Here's how the part is built. I have some questions about the finished solid (model axes, mm). A direction names the side the tool comes from. Coordinates: 2 decimals unless noted, no trailing zeros. Order: outer loops, then holes, each group sorted by start corner. A loop starts at its lowest first (then second) coordinate and runs counter-clockwise, first axis right, second up. Notation, with made-up numbers: (43.25, -30) -> (72.25, -30) arc R15 ccw to (72.25, -9) -> close; hole circle Ø5 at (7, 15.5). An arc over 180 degrees is marked (long way). One line per item, written item: value. Start each with the question number.
```python
from build123d import *

# Parameters (mm, degrees)
F1_DEPTH = 1.5
F2_DEPTH = 14
F4_W     = 26.8
F4_H     = 15.749622
F5_DEPTH = 26
F6_R     = 3
F7_R     = 0.7
F9_DEPTH = 18.8


with BuildPart() as f1:
    # F0 (on Top) → F1 (new body)
    with BuildSketch(Plane.XY):
        Polygon((0, -17.666918), (15.3, -8.833459), (15.3, 8.833459), (0, 17.666918), (-15.3, 8.833459), (-15.3, -8.833459), align=None)
        with BuildLine():
            ThreePointArc((-6.22254, -8.626703), (-8.626703, -8.626703), (-8.626703, -6.22254))
            Line((-8.626703, -6.22254), (-6.505382, -4.101219))
            ThreePointArc((-6.505382, -4.101219), (-4.101219, -4.101219), (-4.101219, -6.505382))
            Line((-4.101219, -6.505382), (-6.22254, -8.626703))
        make_face(mode=Mode.SUBTRACT)
        with BuildLine():
            ThreePointArc((8.626703, -6.22254), (8.626703, -8.626703), (6.22254, -8.626703))
            Line((6.22254, -8.626703), (4.101219, -6.505382))
            ThreePointArc((4.101219, -6.505382), (4.101219, -4.101219), (6.505382, -4.101219))
            Line((6.505382, -4.101219), (8.626703, -6.22254))
        make_face(mode=Mode.SUBTRACT)
        with BuildLine():
            ThreePointArc((-8.626703, 6.22254), (-8.626703, 8.626703), (-6.22254, 8.626703))
            Line((-6.22254, 8.626703), (-4.101219, 6.505382))
            ThreePointArc((-4.101219, 6.505382), (-4.101219, 4.101219), (-6.505382, 4.101219))
            Line((-6.505382, 4.101219), (-8.626703, 6.22254))
        make_face(mode=Mode.SUBTRACT)
        with BuildLine():
            Line((4.101219, 6.505382), (6.22254, 8.626703))
            ThreePointArc((6.22254, 8.626703), (8.626703, 8.626703), (8.626703, 6.22254))
            Line((8.626703, 6.22254), (6.505382, 4.101219))
            ThreePointArc((6.505382, 4.101219), (4.101219, 4.101219), (4.101219, 6.505382))
        make_face(mode=Mode.SUBTRACT)
    extrude(amount=F1_DEPTH)

    # F0 (on Top) → F2 (join)
    with BuildSketch(Plane.XY):
        Polygon((-17.8, 10.276835), (-17.8, -10.276835), (0, -20.55367), (17.8, -10.276835), (17.8, 10.276835), (0, 20.55367), align=None)
        Polygon((15.3, 8.833459), (15.3, -8.833459), (0, -17.666918), (-15.3, -8.833459), (-15.3, 8.833459), (0, 17.666918), align=None, mode=Mode.SUBTRACT)
    extrude(amount=F2_DEPTH)

    # F4 (on offset) → F5 (cut)
    with BuildSketch(Plane.XZ.offset(-25)):
        with Locations((0, 9.374811)):
            Rectangle(F4_W, F4_H)
    extrude(amount=F5_DEPTH, mode=Mode.SUBTRACT)

    # F6
    f6_edges = [f1.edges().sort_by_distance(p)[0] for p in [
        (17.8, 10.276835, 7),
        (-17.8, 10.276835, 7),
        (-17.8, -10.276835, 7),
        (0, -20.55367, 7),
        (17.8, -10.276835, 7),
        (15.3, 8.833459, 7.75),
        (15.3, -8.833459, 7.75),
        (0, -17.666918, 7.75),
        (-15.3, -8.833459, 7.75),
        (-15.3, 8.833459, 7.75),
    ]]
    fillet(f6_edges, radius=F6_R)

    # F7
    f7_edges = [f1.edges().sort_by_distance(p)[0] for p in [
        (-13.6, 9.814955, 1.5),
        (0, 20.55367, 0.75),
    ]]
    fillet(f7_edges, radius=F7_R)

    # F8 (on Right) → F9 (cut, symmetric)
    with BuildSketch(Plane.YZ):
        with BuildLine():
            Line((13.07399, 14), (-7.101408, 14))
            add(Edge.make_bspline(
                [(-7.101408, 14), (4.434353, 14), (10.286969, 11.588226), (13.07399, 6.5)],
                knots=[0, 0, 0, 0, 21.524328, 21.524328, 21.524328, 21.524328], degree=3))
            Line((13.07399, 6.5), (13.07399, 14))
        make_face()
    extrude(amount=F9_DEPTH, both=True, mode=Mode.SUBTRACT)


solid = f1.part
```
Q1. Imagine slicing it at A-A (z = 5.25). Write out the boundary of the cut face in (x, y).
Q2. Imagine slicing it at D-D (y = 16). Write out the boundary of the cut face in (x, z), plus the area to 3 significant figures.
Q3. If we mould it in two halves opening along X, with no side actions, what happens to faces 6 (the face through (5.177, -7.581, 0.74)), 7 (the face through (-17.409, -10.026, 7.098)), 8 (the face through (4.1, 4.1, 0.7)), 9 (the face through (8.796, -15.475, 6.902))? For each: +X half, -X half, draft (parallel to the pull), parting line (faces both ways), or undercut.
Q4. For faces 1 (the face through (13.4, 11, 5)), 2 (the face through (-17.8, 0, 7)), 3 (the face through (14.9, 8.6, 7.1)), 4 (the face through (17.39, 10.06, 5.62)), 5 (the face through (5.147, 7.551, 0.74)), which set-ups out of +Z, -Z, +X, -X, +Y, -Y let a thin tool reach every point of the face, with its end or its side?
Q5. For P1, Ø2, axis at x = 11.5, z = 4, coming from the +Y side; P2, Ø3, axis at x = 4.5, y = -13, coming from the +Z side; P3, Ø6, axis at x = 11, y = -1, coming from the -Z side; P4, Ø3, axis at x = 3, z = 9, coming from the -Y side, each with a flat end and sliding along its axis, tell me the tip position at first contact or that it passes through.
Q6. Imagine slicing it at B-B (x = 5.5). Count the separate pieces of the cut face and the enclosed holes in it, plus the area to 3 significant figures.
Q7. I need wall thicknesses on line 1 (X direction, y = 0, z = 11.5); line 2 (Z direction, x = -11, y = -8); line 3 (X direction, y = 9.5, z = 2.5). Which ranges of each line are inside material? Lowest first, please.
Completed:
1. outline: (-17.8, -8.54) arc R3 ccw to (-16.3, -11.14) -> (-1.5, -19.69) arc R3 ccw to (1.5, -19.69) -> (16.3, -11.14) arc R3 ccw to (17.8, -8.54) -> (17.8, 8.54) arc R3 ccw to (16.3, 11.14) -> (13.4, 12.82) -> (13.4, 9.93) -> (13.8, 9.7) arc R3 cw to (15.3, 7.1) -> (15.3, -7.1) arc R3 cw to (13.8, -9.7) -> (1.5, -16.8) arc R3 cw to (-1.5, -16.8) -> (-13.8, -9.7) arc R3 cw to (-15.3, -7.1) -> (-15.3, 7.1) arc R3 cw to (-13.8, 9.7) -> (-13.4, 9.93) -> (-13.4, 12.82) -> (-16.3, 11.14) arc R3 ccw to (-17.8, 8.54) -> close
2. outline: (-7.89, 0) -> (7.89, 0) -> (7.89, 1.5) -> (-7.89, 1.5) -> close
2. area: 23.7 mm2
3. face 6: undercut
3. face 7: -X half
3. face 8: undercut
3. face 9: +X half
4. face 1: +Z, +Y
4. face 2: +Z, -Z, -X, +Y, -Y
4. face 3: +Z
4. face 4: +Z, -Z, +X, +Y
4. face 5: +Z, -Z
5. P1: stops at y = -10.45
5. P2: stops at z = 1.63
5. P3: stops at z = 0
5. P4: stops at y = -19.69
6. separate pieces: 3
6. enclosed holes: 0
6. area: 75.5 mm2
7. line 1: x = -17.8 to -15.3, 15.3 to 17.8
7. line 2: z = 0 to 1.5
7. line 3: x = -17.64 to -14.1, 14.1 to 17.64
